```python
from build123d import *

# Parameters (mm, degrees)
SKETCH2_W                = 15
SKETCH2_H                = 36
BOSS_EXTRUDE1_DEPTH      = 8
SKETCH4_R                = 4.1
CUT_EXTRUDE1_DEPTH       = 22.077238908
CUT_EXTRUDE2_DEPTH       = 2.4
CUT_EXTRUDE5_DEPTH       = 2.4
CUT_EXTRUDE8_DEPTH       = 2.4
CUT_EXTRUDE9_REACH       = 25.383
CUT_EXTRUDE9_END_RADIUS  = 4.1
SKETCH21_R               = 1.6
CUT_EXTRUDE10_REACH      = 25.383
CUT_EXTRUDE10_END_RADIUS = 4.1
SKETCH16_R               = 1.6
SKETCH24_R               = 1.6
CUT_EXTRUDE11_DEPTH      = 24.382899769


with BuildPart() as part:
    # Sketch2 → Boss-Extrude1 (new body)
    with BuildSketch(Plane(origin=(0, 0, 0), x_dir=(1, 0, 0), z_dir=(0, 1, 0))):
        Rectangle(SKETCH2_W, SKETCH2_H)
    extrude(amount=BOSS_EXTRUDE1_DEPTH)

    # Sketch4 → Cut-Extrude1 (cut, through all)
    with BuildSketch(Plane(origin=(0, 8, 0), x_dir=(1, 0, 0), z_dir=(0, 1, 0))):
        with Locations(Location((0, 0, 0), (0, 0, 270))):
            Circle(SKETCH4_R)
    extrude(amount=-CUT_EXTRUDE1_DEPTH, mode=Mode.SUBTRACT)

    # Sketch13 → Cut-Extrude2 (cut)
    with BuildSketch(Plane.ZY.offset(7.5)):
        Polygon((16.3, 4), (14.75, 6.684678752), (11.65, 6.684678752), (10.1, 4), (11.65, 1.315321248), (14.75, 1.315321248), align=None)
        Polygon((-10.1, 4), (-11.65, 6.684678752), (-14.75, 6.684678752), (-16.3, 4), (-14.75, 1.315321248), (-11.65, 1.315321248), align=None)
    extrude(amount=-CUT_EXTRUDE2_DEPTH, mode=Mode.SUBTRACT)

    # Sketch15 → Cut-Extrude5 (cut)
    with BuildSketch(Plane(origin=(7.5, 0, 0), x_dir=(0, 0, -1), z_dir=(1, 0, 0))):
        Polygon((-3.1, 4), (-1.55, 1.315321248), (1.55, 1.315321248), (3.1, 4), (1.55, 6.684678752), (-1.55, 6.684678752), align=None)
    extrude(amount=-CUT_EXTRUDE5_DEPTH, mode=Mode.SUBTRACT)

    # Sketch20 → Cut-Extrude8 (cut)
    with BuildSketch(Plane.ZY.offset(7.5)):
        Polygon((3.1, 4), (1.55, 6.684678752), (-1.55, 6.684678752), (-3.1, 4), (-1.55, 1.315321248), (1.55, 1.315321248), align=None)
    extrude(amount=-CUT_EXTRUDE8_DEPTH, mode=Mode.SUBTRACT)

    # Cut-Extrude9: up to this cylinder (the profile starts outside it)
    cut_extrude9_end = Plane(origin=(0, 4, 0), z_dir=(0, 1, 0)) * Cylinder(CUT_EXTRUDE9_END_RADIUS, 59.966, mode=Mode.PRIVATE)
    # Sketch21 → Cut-Extrude9 (cut, up to the surface)
    with BuildSketch(Plane.ZY.offset(5.1), mode=Mode.PRIVATE) as cut_extrude9_sk1:
        with Locations((0, 4)):
            Circle(SKETCH21_R)
    cut_extrude9_tool1 = extrude(cut_extrude9_sk1.sketch, amount=-CUT_EXTRUDE9_REACH, mode=Mode.PRIVATE) - cut_extrude9_end
    add(cut_extrude9_tool1.solids().sort_by_distance((-5.1, 4, 0))[0], mode=Mode.SUBTRACT)

    # Cut-Extrude10: up to this cylinder (the profile starts outside it)
    cut_extrude10_end = Plane(origin=(0, 4, 0), z_dir=(0, 1, 0)) * Cylinder(CUT_EXTRUDE10_END_RADIUS, 59.966, mode=Mode.PRIVATE)
    # Sketch16 → Cut-Extrude10 (cut, up to the surface)
    with BuildSketch(Plane(origin=(5.1, 0, 0), x_dir=(0, 0, -1), z_dir=(1, 0, 0)), mode=Mode.PRIVATE) as cut_extrude10_sk1:
        with Locations(Location((0, 4, 0), (0, 0, 180))):
            Circle(SKETCH16_R)
    cut_extrude10_tool1 = extrude(cut_extrude10_sk1.sketch, amount=-CUT_EXTRUDE10_REACH, mode=Mode.PRIVATE) - cut_extrude10_end
    add(cut_extrude10_tool1.solids().sort_by_distance((5.1, 4, 0))[0], mode=Mode.SUBTRACT)

    # Sketch24 → Cut-Extrude11 (cut, through all)
    with BuildSketch(Plane.ZY.offset(5.1)):
        with Locations((13.147013408, 4)):
            Circle(SKETCH24_R)
        with Locations((-13.252986592, 4)):
            Circle(SKETCH24_R)
    extrude(amount=-CUT_EXTRUDE11_DEPTH, mode=Mode.SUBTRACT)


solid = part.part
```
The model under review builds one solid part; all positions refer to its coordinate system, in mm. A direction names the side the tool comes from. Coordinates: 2 decimals unless noted, no trailing zeros. Write each loop counter-clockwise with the first axis right and the second up, starting at its lowest first coordinate (ties: lowest second). Pieces come first, ordered by that corner, then holes. Notation, with made-up numbers: (36, -11.5) - (78, -11.5) arc R16 ccw to (78, -1.5) - close; hole circle Ø1 at (0, 36.25). An arc over 180 degrees is marked (long way). Write item = value, one per line.
(1) For line 1 (Z direction, x = 4.5, y = 5.25); line 2 (Z direction, x = -0.75, y = 4.5); line 3 (Y direction, x = -4.6, z = 0), list the stretches that pass through material, from the lowest coordinate up. Write a range as [from, to].
Result sheet:
line_1 = [-18, -14.25], [-12.25, -1], [1, 12.15], [14.15, 18]
line_2 = [-18, -14.77], [-11.73, -4.03], [4.03, 11.63], [14.67, 18]
line_3 = [0, 2.4], [5.6, 8]
(2) For P1, Ø2.5, axis at y = 4.5, z = 0, coming from the +X side; P2, Ø3.5, axis at y = 4, z = 0, coming from the -X side, all flat-tipped, find the tip position at first contact; note any pin that passes through.
Result sheet:
P1 = 5.1
P2 = -5.1
(3) Machinability: for faces 1 (the face through (1.11, 4.07, 11.55)), 2 (the face through (6.317, 5.361, 2.314)), 3 (the face through (-6.317, 2.639, 2.314)), which of the approach directions +Z, -Z, +X, -X, +Y, -Y give a long, thin tool a straight path to every point of the face, cutting with its end or side? Answer none if there is none.
Result sheet:
face_1 = +X, -X
face_2 = +X
face_3 = -X
(4) Mouldability with a two-part tool opening along Z and no side actions: class faces 4 (the face through (-0.1, 0, -4.3)), 5 (the face through (-6.317, 2.639, 15.514)) as pulls with the +Z half, pulls with the -Z half, needs draft (parallel to the pull), parting line crosses it, or undercut.
Result sheet:
face_4 = needs draft
face_5 = undercut
(5) Consider section C-C, the plane x = 6. Give the boundary of the cut face in (y, z).
Result sheet:
outline = (0, -18) - (8, -18) - (8, 18) - (0, 18) - close; hole (1.32, -1.55) - (4, -3.1) - (6.68, -1.55) - (6.68, 1.55) - (4, 3.1) - (1.32, 1.55) - close; hole circle Ø3.2 at (4, -13.25); hole circle Ø3.2 at (4, 13.15)
(6) Consider section B-B, the plane z = 0. Give the boundary of the cut face in (x, y), then the cut area to 3 significant figures.
Result sheet:
outline = (-7.5, 0) - (-4.1, 0) - (-4.1, 2.4) - (-5.1, 2.4) - (-5.1, 1.32) - (-7.5, 1.32) - close; (-7.5, 6.68) - (-5.1, 6.68) - (-5.1, 5.6) - (-4.1, 5.6) - (-4.1, 8) - (-7.5, 8) - close; (4.1, 0) - (7.5, 0) - (7.5, 1.32) - (5.1, 1.32) - (5.1, 2.4) - (4.1, 2.4) - close; (4.1, 5.6) - (5.1, 5.6) - (5.1, 6.68) - (7.5, 6.68) - (7.5, 8) - (4.1, 8) - close
area = 22.2 mm^2
(7) Consider section A-A, the plane x = 0. Give the boundary of the cut face in (y, z), then the cut area to 3 significant figures.
Result sheet:
outline = (0, -18) - (8, -18) - (8, -4.1) - (0, -4.1) - close; (0, 4.1) - (8, 4.1) - (8, 18) - (0, 18) - close; hole circle Ø3.2 at (4, -13.25); hole circle Ø3.2 at (4, 13.15)
area = 206 mm^2
(8) Consider section D-D, the plane x = 2.5. Give the boundary of the cut face in (y, z), then the cut area to 3 significant figures.
Result sheet:
outline = (0, -18) - (8, -18) - (8, -3.25) - (0, -3.25) - close; (0, 3.25) - (8, 3.25) - (8, 18) - (0, 18) - close; hole circle Ø3.2 at (4, -13.25); hole circle Ø3.2 at (4, 13.15)
area = 220 mm^2
